from build123d import *

# Parameters (mm, degrees)
F1_DEPTH = 25
F1_TAPER = 10
F4_DEPTH = 20
F5_DEPTH = 20
F6_T     = -0.7
F7_R     = 1


with BuildPart() as f1:
    # F0 (on Top) → F1 (new body)
    with BuildSketch(Plane.XY):
        with BuildLine():
            ThreePointArc((40, 15), (37.0710678119, 22.0710678119), (30, 25))
            Line((30, 25), (-30, 25))
            ThreePointArc((-30, 25), (-37.0710678119, 22.0710678119), (-40, 15))
            Line((-40, 15), (-40, -15))
            ThreePointArc((-40, -15), (-37.0710678119, -22.0710678119), (-30, -25))
            Line((-30, -25), (30, -25))
            ThreePointArc((30, -25), (37.0710678119, -22.0710678119), (40, -15))
            Line((40, -15), (40, 15))
        make_face()
    extrude(amount=F1_DEPTH, taper=F1_TAPER)

    # F2 (on face) → F4 (cut)
    with BuildSketch(Plane.XY.offset(25)):
        with BuildLine():
            Line((20.3824352339, 17.5), (14.3824352339, 17.5))
            ThreePointArc((14.3824352339, 17.5), (13.6753284527, 17.2071067812), (13.3824352339, 16.5))
            Line((13.3824352339, 16.5), (13.3824352339, 13.5))
            ThreePointArc((13.3824352339, 13.5), (13.0895420151, 12.7928932188), (12.3824352339, 12.5))
            Line((12.3824352339, 12.5), (5.8824352339, 12.5))
            ThreePointArc((5.8824352339, 12.5), (5.1753284527, 12.2071067812), (4.8824352339, 11.5))
            Line((4.8824352339, 11.5), (4.8824352339, -11.5))
            ThreePointArc((4.8824352339, -11.5), (5.1753284527, -12.2071067812), (5.8824352339, -12.5))
            Line((5.8824352339, -12.5), (12.3824352339, -12.5))
            ThreePointArc((12.3824352339, -12.5), (13.0895420151, -12.7928932188), (13.3824352339, -13.5))
            Line((13.3824352339, -13.5), (13.3824352339, -16.5))
            ThreePointArc((13.3824352339, -16.5), (13.6753284527, -17.2071067812), (14.3824352339, -17.5))
            Line((14.3824352339, -17.5), (20.3824352339, -17.5))
            ThreePointArc((20.3824352339, -17.5), (21.0895420151, -17.2071067812), (21.3824352339, -16.5))
            Line((21.3824352339, -16.5), (21.3824352339, -13.5))
            ThreePointArc((21.3824352339, -13.5), (21.6753284527, -12.7928932188), (22.3824352339, -12.5))
            Line((22.3824352339, -12.5), (28.8824352339, -12.5))
            ThreePointArc((28.8824352339, -12.5), (29.5895420151, -12.2071067812), (29.8824352339, -11.5))
            Line((29.8824352339, -11.5), (29.8824352339, 11.5))
            ThreePointArc((29.8824352339, 11.5), (29.5895420151, 12.2071067812), (28.8824352339, 12.5))
            Line((28.8824352339, 12.5), (22.3824352339, 12.5))
            ThreePointArc((22.3824352339, 12.5), (21.6753284527, 12.7928932188), (21.3824352339, 13.5))
            Line((21.3824352339, 13.5), (21.3824352339, 16.5))
            ThreePointArc((21.3824352339, 16.5), (21.0895420151, 17.2071067812), (20.3824352339, 17.5))
        make_face()
    extrude(amount=-F4_DEPTH, mode=Mode.SUBTRACT)

    # F3 (on face) → F5 (cut)
    with BuildSketch(Plane.XY.offset(25)):
        with BuildLine():
            Line((-11.9747403339, 12.5), (-17.9747403339, 12.5))
            ThreePointArc((-17.9747403339, 12.5), (-18.681847115, 12.2071067812), (-18.9747403339, 11.5))
            Line((-18.9747403339, 11.5), (-18.9747403339, -11.5))
            ThreePointArc((-18.9747403339, -11.5), (-18.681847115, -12.2071067812), (-17.9747403339, -12.5))
            Line((-17.9747403339, -12.5), (-11.9747403339, -12.5))
            ThreePointArc((-11.9747403339, -12.5), (-11.2676335527, -12.2071067812), (-10.9747403339, -11.5))
            Line((-10.9747403339, -11.5), (-10.9747403339, 11.5))
            ThreePointArc((-10.9747403339, 11.5), (-11.2676335527, 12.2071067812), (-11.9747403339, 12.5))
        make_face()
    extrude(amount=-F5_DEPTH, mode=Mode.SUBTRACT)

    # F6
    f6_openings = [f1.faces().sort_by_distance(p)[0] for p in [
        (0, 0, 0),
    ]]
    offset(amount=F6_T, openings=f6_openings, kind=Kind.INTERSECTION)

    # F7
    f7_edges = [f1.edges().sort_by_distance(p)[0] for p in [
        (33.954018, 18.954018, 25),
        (35.591825, 0, 25),
        (0, 20.591825, 25),
        (33.954018, -18.954018, 25),
        (-33.954018, 18.954018, 25),
        (0, -20.591825, 25),
        (-35.591825, 0, 25),
        (-33.954018, -18.954018, 25),
        (-11.267634, 12.207107, 25),
        (-14.97474, 12.5, 25),
        (-18.681847, 12.207107, 25),
        (-18.97474, 0, 25),
        (-18.681847, -12.207107, 25),
        (-14.97474, -12.5, 25),
        (-11.267634, -12.207107, 25),
        (-10.97474, 0, 25),
        (21.382435, 15, 25),
        (21.675328, 12.792893, 25),
        (21.089542, 17.207107, 25),
        (25.632435, 12.5, 25),
        (17.382435, 17.5, 25),
        (29.589542, 12.207107, 25),
        (13.675328, 17.207107, 25),
        (29.882435, 0, 25),
        (13.382435, 15, 25),
        (29.589542, -12.207107, 25),
        (13.089542, 12.792893, 25),
        (25.632435, -12.5, 25),
        (9.132435, 12.5, 25),
        (21.675328, -12.792893, 25),
        (5.175328, 12.207107, 25),
        (21.382435, -15, 25),
        (4.882435, 0, 25),
        (21.089542, -17.207107, 25),
        (5.175328, -12.207107, 25),
        (17.382435, -17.5, 25),
        (9.132435, -12.5, 25),
        (13.675328, -17.207107, 25),
        (13.089542, -12.792893, 25),
        (13.382435, -15, 25),
    ]]
    fillet(f7_edges, radius=F7_R)


solid = f1.part
Check sheet for the modelled part. Datum: model origin and axes. Units: mm. A direction names the side the tool comes from. Round coordinates to 2 decimals unless told otherwise and drop trailing zeros. Order: outer loops, then holes, each group sorted by start corner. A loop starts at its lowest first (then second) coordinate and runs counter-clockwise, first axis right, second up.
Q1. Cross-section at A-A, the plane x = -7.5. Enter the section's corners in (y, z), plus the area to 3 significant figures.
Filled sheet:
outline: (-25, 0) - (-24.29, 0) - (-20, 24.3) - (20, 24.3) - (24.29, 0) - (25, 0) - (20.74, 24.17) arc R1 ccw to (19.75, 25) - (-19.75, 25) arc R1 ccw to (-20.74, 24.17) - close
area: 63.2 mm2
Q2. Scan lines: L1, parallel to X at y = -15.5, z = 16.75; L2, parallel to Y at x = -12, z = 20; L3, parallel to Y at x = 19, z = 9. Record each from-to range of solid material in increasing order.
Filled sheet:
L1: x = -37.03 to -36.32, 12.68 to 13.38, 21.38 to 22.08, 36.32 to 37.03
L2: y = -21.47 to -20.76, -13.2 to -12.5, 12.5 to 13.2, 20.76 to 21.47
L3: y = -23.41 to -22.7, -18.2 to -17.5, 17.5 to 18.2, 22.7 to 23.41
Q3. Draft check along X on faces 1 (the face through (-37.9, -0.2, 11.9)), 2 (the face through (35.482, -20.604, 12.256)), 3 (the face through (-15, -12.5, 15)). Enter one of: pulls with the +X half, pulls with the -X half, needs draft (parallel to the pull), parting line crosses it, or undercut.
Filled sheet:
face 1: pulls with the -X half
face 2: pulls with the +X half
face 3: undercut
Q4. Set-up check for faces 4 (the face through (12.682, -15, 14)), 5 (the face through (-35.482, 20.604, 12.256)), 6 (the face through (-10.975, 0, 15)): record each of +Z, -Z, +X, -X, +Y, -Y from which the full face is reachable in a straight line by a thin tool's end or side.
Filled sheet:
face 4: -Z
face 5: +Z, -X, +Y
face 6: +Z
Q5. Depth check by flat-ended pin: P1, Ø12.5, axis at x = 14, y = -3.5, coming from the +Z side; P2, Ø5, axis at x = 27, z = 10.5, coming from the -Y side; P3, Ø0.9, axis at y = -14.5, z = 10, coming from the -X side. Enter the tip coordinate at first touch or a pass-through.
Filled sheet:
P1: stops at z = 5
P2: stops at y = -23.59
P3: stops at x = -38.32
Q6. Cross-section at B-B, the plane z = 7.5. Give the number of separate pieces and of enclosed holes in the cut face, plus the area to 3 significant figures.
Filled sheet:
separate pieces: 3
enclosed holes: 3
area: 294 mm2
Q7. Cross-section at D-D, the plane x = 28. Enter the section's corners in (y, z), plus the area to 3 significant figures.
Filled sheet:
outline: (-25, 0) - (-24.29, 0) - (-20, 24.3) - (-13.2, 24.3) - (-13.2, 4.3) - (13.2, 4.3) - (13.2, 24.3) - (20, 24.3) - (24.29, 0) - (25, 0) - (20.74, 24.17) arc R1 ccw to (19.75, 25) - (13.5, 25) arc R1 ccw to (12.5, 24) - (12.5, 5) - (-12.5, 5) - (-12.5, 24) arc R1 ccw to (-13.5, 25) - (-19.75, 25) arc R1 ccw to (-20.74, 24.17) - close
area: 90.7 mm2
